```python
from build123d import *

# Parameters (mm, degrees)
SKETCH1_W                                         = 112.782
SKETCH1_H                                         = 3.175
BOSS_EXTRUDE1_DEPTH                               = 99.75
BOSS_EXTRUDE1_DEPTH_BACK                          = 35
SKETCH2_R                                         = 3.175
CUT_EXTRUDE1_DEPTH                                = 15.975
CUT_EXTRUDE1_DEPTH_BACK                           = 1
M4_CLEARANCE_HOLE1_D                              = 4.3
CSK_FOR_4_FLAT_HEAD_MACHINE_SCREW_100_D           = 2.9464
CSK_FOR_4_FLAT_HEAD_MACHINE_SCREW_100_CSINK_D     = 5.715
CSK_FOR_4_FLAT_HEAD_MACHINE_SCREW_100_CSINK_ANGLE = 100
SKETCH8_R                                         = 3
CUT_EXTRUDE3_DEPTH                                = 3.5
F_6_32_TAPPED_HOLE1_D                             = 2.7051
F_1_4_20_TAPPED_HOLE1_D                           = 5.1054
SKETCH16_R                                        = 2.9972
CUT_EXTRUDE4_DEPTH                                = 4.175


with BuildPart() as part:
    # Sketch1 → Boss-Extrude1 (new body, two sides)
    with BuildSketch(Plane(origin=(0, 0, 0), x_dir=(1, 0, 0), z_dir=(0, 1, 0))) as boss_extrude1_sk:
        with Locations((23.753, -13.3875)):
            Rectangle(SKETCH1_W, SKETCH1_H)
    extrude(amount=BOSS_EXTRUDE1_DEPTH)
    extrude(boss_extrude1_sk.sketch, amount=-BOSS_EXTRUDE1_DEPTH_BACK)

    # Sketch2 → Cut-Extrude1 (cut, two sides)
    with BuildSketch(Plane.XY) as cut_extrude1_sk:
        with Locations((52.316, 28.127026218)):
            Circle(SKETCH2_R)
        with Locations((67.816, 28.127026218)):
            Circle(SKETCH2_R)
        Polygon((48, -35), (80.144, -35), (80.144, 8.487287802), (48, -14.020183306), align=None)
        with BuildLine():
            Line((60.066, 56.550419976), (80.066, 56.550419976))
            ThreePointArc((80.066, 56.550419976), (88.066, 48.550419976), (80.066, 40.550419976))
            Line((80.066, 40.550419976), (60.066, 40.550419976))
            ThreePointArc((60.066, 40.550419976), (52.066, 48.550419976), (60.066, 56.550419976))
        make_face()
        Polygon((43.964687276, 99.75), (80.144, 74.416972504), (80.144, 99.75), align=None)
    extrude(amount=CUT_EXTRUDE1_DEPTH, mode=Mode.SUBTRACT)
    extrude(cut_extrude1_sk.sketch, amount=-CUT_EXTRUDE1_DEPTH_BACK, mode=Mode.SUBTRACT)

    # M4 Clearance Hole1 (through all)
    with Locations(Plane.XY.offset(14.975)):
        with Locations((-13.356, 28), (31.644, 28), (31.644, -28), (-13.356, -28)):
            Hole(M4_CLEARANCE_HOLE1_D / 2)

    # CSK for #4 Flat Head Machine Screw (100)1 (through all)
    with Locations(Plane.XY.offset(14.975)):
        with Locations((19.352, 96.519071488), (28.871071488, 87), (19.352, 77.480928512)):
            CounterSinkHole(CSK_FOR_4_FLAT_HEAD_MACHINE_SCREW_100_D / 2, CSK_FOR_4_FLAT_HEAD_MACHINE_SCREW_100_CSINK_D / 2, counter_sink_angle=CSK_FOR_4_FLAT_HEAD_MACHINE_SCREW_100_CSINK_ANGLE)

    # Sketch8 → Cut-Extrude3 (cut)
    with BuildSketch(Plane.XY.offset(14.975)):
        with Locations((19.352, 87)):
            Circle(SKETCH8_R)
    extrude(amount=-CUT_EXTRUDE3_DEPTH, mode=Mode.SUBTRACT)

    # #6-32 Tapped Hole1 (through all)
    with Locations(Plane.XY.offset(14.975)):
        with Locations((-28.824, -3.758), (-21.077, 4.878), (-28.824, 13.514)):
            Hole(F_6_32_TAPPED_HOLE1_D / 2)

    # 1/4-20 Tapped Hole1 (through all)
    with Locations(Plane.XY.offset(14.975)):
        with Locations((57.526, 13.97), (71.75, 13.97), (71.75, 69.85), (57.526, 69.85)):
            Hole(F_1_4_20_TAPPED_HOLE1_D / 2)

    # Sketch16 → Cut-Extrude4 (cut, through all)
    with BuildSketch(Plane.XY.offset(14.975)):
        with Locations((-14.5061, 86.034)):
            Circle(SKETCH16_R)
    extrude(amount=-CUT_EXTRUDE4_DEPTH, mode=Mode.SUBTRACT)


solid = part.part
```
The listing builds one solid part. Answer for the finished solid, in the listing's coordinates (mm). A direction names the side the tool comes from. Coordinates: 2 decimals unless noted, no trailing zeros. Loops run counter-clockwise (first coordinate to the right, second up) from the corner with the lowest first, then second, coordinate; pieces in that order, holes last. Notation, with made-up numbers: M 46,39.25 L 61,39.25 A33 cw 61,78.25 Z; hole C 82.25,-14.5 d3. An arc over 180 degrees is marked long. Answer as CSV lines item,"result". Start each with the question number.
(1) The part is cut by section C-C (y = -28). Give the vertices of the cut face in (x, z) (3 decimals).
(2) The part is cut by section B-B (z = 12.9). State how many separate pieces and enclosed holes the cut face has, and give its area (3 significant figures).
(3) Given pin 1 (4 mm diameter, centred on x = 28.87, y = 87, fed in from +Z), flat-ended and moving along its own axis, determine where the tip first touches the part or whether it passes through.
(4) For faces 4 (the cylindrical face through (19.54, 97.98, 12.79)), 5 (the flat face through (70, 40.55, 13)), 6 (the flat face through (48, -24, 13)), determine the directions among +Z, -Z, +X, -X, +Y, -Y from which every point of the face is accessible in a straight line to the end or side of a thin tool.
(5) The part is cut by section A-A (y = 69.85). Give the vertices of the cut face in (x, z) (3 decimals).
(6) Find the intervals of material crossed by L1, parallel to Y at x = 54, z = 14.35; L2, parallel to Y at x = 30, z = 12.15; L3, parallel to Y at x = 71.5, z = 12.4, in increasing order. Write a range as [from, to].
(7) The mould has two halves that part along Y. Classify faces 1 (the flat face through (5, 99.75, 13)), 2 (the cylindrical face through (-14.896, 89.006, 13.41)), 3 (the flat face through (23, 33, 11.8)): pulls with the +Y half, pulls with the -Y half, needs draft (parallel to the pull), parting line crosses it, or undercut.
Determined:
1,outline,"M -32.638,11.8 L -15.506,11.8 L -15.506,14.975 L -32.638,14.975 Z; M -11.206,11.8 L 29.494,11.8 L 29.494,14.975 L -11.206,14.975 Z; M 33.794,11.8 L 48,11.8 L 48,14.975 L 33.794,14.975 Z"
2,separate pieces,"1"
2,enclosed holes,"18"
2,area,"13,000 mm2"
3,pin 1,"z = 14.26"
4,face 4,"+Z, -Z"
4,face 5,"+Z, -Z, +X"
4,face 6,"+Z, -Z, +X, -Y"
5,outline,"M -32.638,11.8 L 54.973,11.8 L 54.973,14.975 L -32.638,14.975 Z; M 60.079,11.8 L 69.197,11.8 L 69.197,14.975 L 60.079,14.975 Z; M 74.303,11.8 L 80.144,11.8 L 80.144,14.975 L 74.303,14.975 Z"
6,L1,"[-9.82, 25.44], [30.82, 43.33], [53.77, 92.72]"
6,L2,"[-35, -29.39], [-26.61, 26.61], [29.39, 86.05], [87.95, 99.75]"
6,L3,"[2.43, 11.43], [16.51, 40.55], [56.55, 67.31], [72.39, 80.47]"
7,face 1,"pulls with the +Y half"
7,face 2,"undercut"
7,face 3,"needs draft"
